```python
from build123d import *

# Parameters (mm, degrees)
SKETCH1_R             = 12.7
BOSS_EXTRUDE1_DEPTH   = 3.9624
SKETCH2_W             = 7.9121
SKETCH2_H             = 25.4
CUT_EXTRUDE1_DEPTH    = 3.683
SKETCH3_W             = 25.4
SKETCH3_H             = 7.9121
CUT_EXTRUDE2_DEPTH    = 3.683
SKETCH4_W             = 5.44195
SKETCH4_H             = 25.4
CUT_EXTRUDE3_DEPTH    = 1.27
SKETCH5_W             = 25.4
SKETCH5_H             = 5.44195
CUT_EXTRUDE4_DEPTH    = 1.27
CHAMFER1_SIZE         = 2.58492625
CHAMFER1_SIZE2        = 1.492407866
CHAMFER1_PART_2_SIZE  = 2.58492625
CHAMFER1_PART_2_SIZE2 = 1.492407866
CHAMFER1_PART_3_SIZE  = 2.58492625
CHAMFER1_PART_3_SIZE2 = 1.492407866
CHAMFER1_PART_4_SIZE  = 2.58492625
CHAMFER1_PART_4_SIZE2 = 1.492407866
SKETCH6_W             = 8.307705
SKETCH6_H             = 9.2075
CUT_EXTRUDE5_DEPTH    = 3.683
SKETCH7_W             = 9.2075
SKETCH7_H             = 8.307705
CUT_EXTRUDE6_DEPTH    = 3.683


with BuildPart() as part:
    # Sketch1 → Boss-Extrude1 (new body, symmetric)
    with BuildSketch(Plane.XY):
        Circle(SKETCH1_R)
    extrude(amount=BOSS_EXTRUDE1_DEPTH, both=True)

    # Sketch2 → Cut-Extrude1 (cut)
    with BuildSketch(Plane.XY.offset(3.9624)):
        Rectangle(SKETCH2_W, SKETCH2_H)
    extrude(amount=-CUT_EXTRUDE1_DEPTH, mode=Mode.SUBTRACT)

    # Sketch3 → Cut-Extrude2 (cut)
    with BuildSketch(Plane(origin=(0, 0, -3.9624), x_dir=(-1, 0, 0), z_dir=(0, 0, -1))):
        Rectangle(SKETCH3_W, SKETCH3_H)
    extrude(amount=-CUT_EXTRUDE2_DEPTH, mode=Mode.SUBTRACT)

    # Sketch4 → Cut-Extrude3 (cut)
    with BuildSketch(Plane.XY.offset(3.9624)):
        with Locations((9.979025, 0)):
            Rectangle(SKETCH4_W, SKETCH4_H)
        with Locations((-9.979025, 0)):
            Rectangle(SKETCH4_W, SKETCH4_H)
    extrude(amount=-CUT_EXTRUDE3_DEPTH, mode=Mode.SUBTRACT)

    # Sketch5 → Cut-Extrude4 (cut)
    with BuildSketch(Plane(origin=(0, 0, -3.9624), x_dir=(-1, 0, 0), z_dir=(0, 0, -1))):
        with Locations((0, 9.979025)):
            Rectangle(SKETCH5_W, SKETCH5_H)
        with Locations((0, -9.979025)):
            Rectangle(SKETCH5_W, SKETCH5_H)
    extrude(amount=-CUT_EXTRUDE4_DEPTH, mode=Mode.SUBTRACT)

    # Chamfer1
    chamfer1_edges = [part.edges().sort_by_distance(p)[0] for p in [
        (0, 12.7, -2.6924),
    ]]
    chamfer1_side = [part.faces().sort_by_distance(p)[0] for p in [
        (0, 9.480522033, -2.6924),
    ]]
    chamfer(chamfer1_edges, length=CHAMFER1_SIZE, length2=CHAMFER1_SIZE2, reference=chamfer1_side[0])

    # Chamfer1 part 2
    chamfer1_part_2_edges = [part.edges().sort_by_distance(p)[0] for p in [
        (0, -12.7, -2.6924),
    ]]
    chamfer1_part_2_side = [part.faces().sort_by_distance(p)[0] for p in [
        (0, -9.480522033, -2.6924),
    ]]
    chamfer(chamfer1_part_2_edges, length=CHAMFER1_PART_2_SIZE, length2=CHAMFER1_PART_2_SIZE2, reference=chamfer1_part_2_side[0])

    # Chamfer1 part 3
    chamfer1_part_3_edges = [part.edges().sort_by_distance(p)[0] for p in [
        (11.257602653, -5.8784677, 2.6924),
    ]]
    chamfer1_part_3_side = [part.faces().sort_by_distance(p)[0] for p in [
        (9.480522033, 0, 2.6924),
    ]]
    chamfer(chamfer1_part_3_edges, length=CHAMFER1_PART_3_SIZE, length2=CHAMFER1_PART_3_SIZE2, reference=chamfer1_part_3_side[0])

    # Chamfer1 part 4
    chamfer1_part_4_edges = [part.edges().sort_by_distance(p)[0] for p in [
        (-12.7, 0, 2.6924),
    ]]
    chamfer1_part_4_side = [part.faces().sort_by_distance(p)[0] for p in [
        (-9.480522033, 0, 2.6924),
    ]]
    chamfer(chamfer1_part_4_edges, length=CHAMFER1_PART_4_SIZE, length2=CHAMFER1_PART_4_SIZE2, reference=chamfer1_part_4_side[0])

    # Sketch6 → Cut-Extrude5 (cut)
    with BuildSketch(Plane.XY.offset(3.9624)):
        Rectangle(SKETCH6_W, SKETCH6_H)
    extrude(amount=-CUT_EXTRUDE5_DEPTH, mode=Mode.SUBTRACT)

    # Sketch7 → Cut-Extrude6 (cut)
    with BuildSketch(Plane(origin=(0, 0, -3.9624), x_dir=(-1, 0, 0), z_dir=(0, 0, -1))):
        Rectangle(SKETCH7_W, SKETCH7_H)
    extrude(amount=-CUT_EXTRUDE6_DEPTH, mode=Mode.SUBTRACT)


solid = part.part
```
Work out the finished part from the listing and answer in its coordinate system (mm). A direction names the side the tool comes from. Round coordinates to 2 decimals unless told otherwise and drop trailing zeros. Loops run counter-clockwise (first coordinate to the right, second up) from the corner with the lowest first, then second, coordinate; pieces in that order, holes last. Notation, with made-up numbers: (5, -9) -> (15, -9) arc R24 ccw to (15, 12) -> close; hole circle Ø7 at (31.25, -21). An arc over 180 degrees is marked (long way). Write each question's results on one line, items separated by ' | '. Start each with the question number.
1. A tool of negligible diameter and unlimited length cuts with its end or side. For faces 1 (the face through (3.956, -8, 2)), 2 (the face through (8, 0, 2.692)), 3 (the face through (-8, -3.956, -2)), from which of +Z, -Z, +X, -X, +Y, -Y can it reach the whole face along a straight path? Write none if from no direction.
2. Section A-A (z = -3) is taken. Determine the outline of the cut face in (x, y).
3. Given pin 1 Ø4 at (y, z) = (9.5, 2) entering from +X; pin 2 Ø1.4 at (x, y) = (-2, -9) entering from -Z; pin 3 Ø6.5 at (x, y) = (5, 0.5) entering from -Z, each flat-ended and moving along its own axis, determine where each tip first touches the part or whether it passes through.
4. Section B-B (x = 0) is taken. Determine the outline of the cut face in (y, z).
5. For a pull along Y with two mould halves and no side action, classify faces 4 (the face through (10.276, -0.138, 2.599)), 5 (the face through (-3.956, -8, 2)), 6 (the face through (-4.154, 0, 2)) as +Y half, -Y half, draft (parallel to the pull), parting line (faces both ways), or undercut.
6. Section D-D (z = 1.5) is taken. Determine the outline of the cut face in (x, y), plus the area to 3 significant figures.
7. Find the intervals of material crossed by probe 1 along Y at (x, z) = (-1.5, -2.75); probe 2 along X at (y, z) = (-8, 2.75); probe 3 along Z at (x, y) = (6, -0.25), in increasing order. Write a range as from..to.
8. Section C-C (y = 0) is taken. Determine the outline of the cut face in (x, z), plus the area to 3 significant figures.
Evaluation:
1) face 1: +Z, +Y, -Y | face 2: +Z, +X, +Y, -Y | face 3: -Z, +X, -X
2) outline: (-12.07, -3.96) arc R12.7 ccw to (-10.42, -7.26) -> (10.42, -7.26) arc R12.7 ccw to (12.07, -3.96) -> (4.6, -3.96) -> (4.6, -4.15) -> (-4.6, -4.15) -> (-4.6, -3.96) -> close; (-12.07, 3.96) -> (-4.6, 3.96) -> (-4.6, 4.15) -> (4.6, 4.15) -> (4.6, 3.96) -> (12.07, 3.96) arc R12.7 ccw to (10.42, 7.26) -> (-10.42, 7.26) arc R12.7 ccw to start
3) pin 1: stops at x = 10.12 | pin 2: stops at z = -2.69 | pin 3: stops at z = -0.28
4) outline: (-12.7, -1.2) -> (-10.12, -2.69) -> (-7.26, -2.69) -> (-7.26, -3.96) -> (-4.15, -3.96) -> (-4.15, -0.28) -> (4.15, -0.28) -> (4.15, -3.96) -> (7.26, -3.96) -> (7.26, -2.69) -> (10.12, -2.69) -> (12.7, -1.2) -> (12.7, 0.28) -> (-12.7, 0.28) -> close
5) face 4: parting line | face 5: draft | face 6: undercut
6) outline: (-7.26, -10.42) arc R12.7 ccw to (-3.96, -12.07) -> (-3.96, -4.6) -> (-4.15, -4.6) -> (-4.15, 4.6) -> (-3.96, 4.6) -> (-3.96, 12.07) arc R12.7 ccw to (-7.26, 10.42) -> (-7.26, 9.78) arc R12.18 ccw to (-7.26, -9.78) -> close; (3.96, -12.07) arc R12.7 ccw to (7.26, -10.42) -> (7.26, -9.78) arc R12.18 ccw to (7.26, 9.78) -> (7.26, 10.42) arc R12.7 ccw to (3.96, 12.07) -> (3.96, 4.6) -> (4.15, 4.6) -> (4.15, -4.6) -> (3.96, -4.6) -> close | area: 281 mm2
7) probe 1: y = -7.26..-4.15, 4.15..7.26 | probe 2: x = -7.26..-3.96, 3.96..7.26 | probe 3: z = -0.28..3.96
8) outline: (-12.7, -0.28) -> (12.7, -0.28) -> (12.7, 1.2) -> (10.12, 2.69) -> (7.26, 2.69) -> (7.26, 3.96) -> (4.15, 3.96) -> (4.15, 0.28) -> (-4.15, 0.28) -> (-4.15, 3.96) -> (-7.26, 3.96) -> (-7.26, 2.69) -> (-10.12, 2.69) -> (-12.7, 1.2) -> close | area: 59.5 mm2
